from build123d import *

# Parameters (mm, degrees)
EXTRUDE_1_DEPTH     = 8
SKETCH_2_R          = 4
CUT_EXTRUDE_1_DEPTH = 142.73566947
SKETCH_3_W          = 75
SKETCH_3_H          = 8
EXTRUDE_2_DEPTH     = 80
SKETCH_5_R          = 4
CUT_EXTRUDE_2_DEPTH = 147.523035732
RIB_1_REACH         = 156.091
SKETCH_6_WALL_W     = 393.151638598
SKETCH_6_WALL_H     = 8
FILLET_2_R          = 10
SKETCH_7_R          = 8
SKETCH_7_R_2        = 4
EXTRUDE_3_DEPTH     = 3
FILLET_3_R          = 1


with BuildPart() as part:
    # Эскиз1 → Бобышка-Вытянуть1 (new body)
    with BuildSketch(Plane.XY):
        Polygon((0, 0), (75, 0), (75, 30), (55, 120), (0, 120), align=None)
    extrude(amount=EXTRUDE_1_DEPTH)

    # Эскиз2 → Вырез-Вытянуть1 (cut, through all)
    with BuildSketch(Plane.XY.offset(8)):
        with Locations((45, 110)):
            Circle(SKETCH_2_R)
        with Locations((0, 10)):
            Circle(SKETCH_2_R)
        with Locations((65, 10)):
            Circle(SKETCH_2_R)
    extrude(amount=-CUT_EXTRUDE_1_DEPTH, mode=Mode.SUBTRACT)

    # Эскиз3 → Бобышка-Вытянуть2 (add)
    with BuildSketch(Plane.XY.offset(8)):
        with Locations((37.5, 26)):
            Rectangle(SKETCH_3_W, SKETCH_3_H)
    extrude(amount=EXTRUDE_2_DEPTH)

    # Эскиз5 → Вырез-Вытянуть2 (cut, through all)
    with BuildSketch(Plane(origin=(0, 30, 0), x_dir=(1, 0, 0), z_dir=(0, 1, 0))):
        with Locations(Location((50, -30.5, 0), (0, 0, 270))):
            Circle(SKETCH_5_R)
        with Locations(Location((50, -65.5, 0), (0, 0, 270))):
            Circle(SKETCH_5_R)
    extrude(amount=-CUT_EXTRUDE_2_DEPTH, mode=Mode.SUBTRACT)

    # Эскиз6 wall → Ребро1 (add, up to next)
    with BuildSketch(Plane(origin=(35, 11, 48), x_dir=(0, -0.265156483021, -0.964205392804), z_dir=(0, 0.964205392804, -0.265156483021)), mode=Mode.PRIVATE) as rib_1_sk1:
        Rectangle(SKETCH_6_WALL_W, SKETCH_6_WALL_H)
    rib_1_tool1 = extrude(rib_1_sk1.sketch, amount=RIB_1_REACH, mode=Mode.PRIVATE) - part.part
    add(rib_1_tool1.solids().sort_by_distance((35, 11, 48))[0])

    # Скругление2
    fillet_2_edges = [part.edges().sort_by_distance(p)[0] for p in [
        (55, 120, 4),
        (75, 0, 4),
        (75, 26, 88),
    ]]
    fillet(fillet_2_edges, radius=FILLET_2_R)

    # Зеркальное отражение1: part across plane


with BuildPart() as part_1:
    add(part.part)
    add(part.part.mirror(Plane(origin=(0, 120, 8), x_dir=(0, 0, 1), z_dir=(1, 0, 0))))

    # Эскиз7 → Бобышка-Вытянуть3 (add)
    with BuildSketch(Plane.XY.offset(8)):
        with Locations((-45, 110)):
            Circle(SKETCH_7_R)
        with Locations(Location((-45, 110, 0), (0, 0, 180))):
            Circle(SKETCH_7_R_2, mode=Mode.SUBTRACT)
        with Locations((45, 110)):
            Circle(SKETCH_7_R)
        with Locations((45, 110)):
            Circle(SKETCH_7_R_2, mode=Mode.SUBTRACT)
    extrude(amount=EXTRUDE_3_DEPTH)

    # Скругление3
    fillet_3_edges = [part_1.edges().sort_by_distance(p)[0] for p in [
        (-53, 110, 8),
        (37, 110, 8),
    ]]
    fillet(fillet_3_edges, radius=FILLET_3_R)


solid = part_1.part
Could you check a few things on this model? Use its own coordinates, in mm. A direction names the side the tool comes from. Give positions to 0.01 mm unless a question says otherwise; leave off trailing zeros. Order: outer loops, then holes, each group sorted by start corner. A loop starts at its lowest first (then second) coordinate and runs counter-clockwise, first axis right, second up. Notation, with made-up numbers: (11, -24) - (37, -24) arc R25 ccw to (37, 4) - close; hole circle Ø9 at (-7, 41). An arc over 180 degrees is marked (long way). Return JSON: item names as keys, results as strings. Group by question number.
Q1. Suppose I cut it at C-C, the plane x = 59. Please give me the cut outline in (y, z), and give its area (3 significant figures).
Q2. Suppose I cut it at A-A, the plane x = 0. Please give me the cut outline in (y, z).
Q3. Suppose I cut it at B-B, the plane z = 67. Please give me the cut outline in (x, y) (3 decimals), and give its area (3 significant figures).
Q4. Please list where these lines run through material, in increasing order: line 1 along X through (y, z) = (27, 30); line 2 along Y through (x, z) = (45, 9); line 3 along X through (y, z) = (14, 21). Write a range as [from, to].
Q5. Which directions (+Z, -Z, +X, -X, +Y, -Y) give clear straight access to the entire face, cutting with the end or side of a thin tool? Please do faces 5 (the face through (-57, 22, 47)), 6 (the face through (-31, 17, 38)), 7 (the face through (57, 22, 47)).
Q6. Suppose I cut it at D-D, the plane z = 20. Please give me the cut outline in (x, y), and give its area (3 significant figures).
Q7. Thinking about a two-plate mould opening in Y: for faces 1 (the face through (-75, 24, 38)), 2 (the face through (66, 70.5, 3.9)), 3 (the face through (1, 0, 4)), 4 (the face through (-44.479, 106.034, 5.423)), which applies, pulls with the +Y half, pulls with the -Y half, needs draft (parallel to the pull), parting line crosses it, or undercut?
Q8. Will these pins go through, and if not, where does the flat tip stop? pin 1 Ø7 at (x, y) = (0, 10) entering from +Z; pin 2 Ø1.5 at (x, z) = (9.5, 52) entering from +Y; pin 3 Ø1 at (x, y) = (-56.5, 83) entering from +Z; pin 4 Ø17.5 at (x, y) = (-43.5, 110) entering from +Z.
Resolved:
{
 "1": {"outline": "(0, 0) - (102, 0) - (102, 8) - (30, 8) - (30, 88) - (22, 88) - (22, 8) - (0, 8) - close", "area": "1,460 mm2"},
 "2": {"outline": "(0, 0) - (6, 0) - (6, 8) - (0, 8) - close; (14, 0) - (120, 0) - (120, 8) - (30, 8) - (30, 88) - (22, 88) - (22, 8) - (14, 8) - close"},
 "3": {"outline": "(-75, 22) - (-53.708, 22) - (-53.708, 30) - (-75, 30) - close; (-46.292, 22) - (-39, 22) - (-39, 16.225) - (-31, 16.225) - (-31, 22) - (31, 22) - (31, 16.225) - (39, 16.225) - (39, 22) - (46.292, 22) - (46.292, 30) - (-46.292, 30) - close; (53.708, 22) - (75, 22) - (75, 30) - (53.708, 30) - close", "area": "1,170 mm2"},
 "4": {"line 1": "x = [-75, -53.97], [-46.03, 46.03], [53.97, 75]", "line 2": "y = [22, 30], [102, 106], [114, 118]", "line 3": "x = [-39, -31], [31, 39]"},
 "5": {"face 5": "+Z, -X, -Y", "face 6": "+Z, -Y", "face 7": "+Z, +X, -Y"},
 "6": {"outline": "(-75, 22) - (-39, 22) - (-39, 3.3) - (-31, 3.3) - (-31, 22) - (31, 22) - (31, 3.3) - (39, 3.3) - (39, 22) - (75, 22) - (75, 30) - (-75, 30) - close", "area": "1,500 mm2"},
 "7": {"face 1": "needs draft", "face 2": "pulls with the +Y half", "face 3": "pulls with the -Y half", "face 4": "undercut"},
 "8": {"pin 1": "passes through", "pin 2": "stops at y = 30", "pin 3": "stops at z = 8", "pin 4": "stops at z = 11"}
}
